```python
from build123d import *

# Parameters (mm, degrees)
SKETCH1_W                   = 15
SKETCH1_H                   = 4.9
SKETCH1_W_2                 = 5
SKETCH1_H_2                 = 19.05
SKETCH1_W_3                 = 14.05
BOSS_EXTRUDE1_DEPTH         = 30
SKETCH2_R                   = 6.4
CUT_EXTRUDE1_DEPTH          = 43.069832248
CUT_EXTRUDE2_DEPTH          = 30
FILLET1_R                   = 2.5
TAP_DRILL_FOR_M5X0_8_TAP1_D = 4.2


with BuildPart() as part:
    # Sketch1 → Boss-Extrude1 (new body)
    with BuildSketch(Plane(origin=(0, 0, 0), x_dir=(1, 0, 0), z_dir=(0, 1, 0))):
        with Locations((2.312030075, 14.354511278)):
            Rectangle(SKETCH1_W, SKETCH1_H)
        Polygon((-5.187969925, 16.804511278), (-10.187969925, 16.804511278), (-10.187969925, 11.329511278), (-5.187969925, 11.329511278), (-5.187969925, 11.904511278), align=None)
        with Locations((-7.687969925, 1.804511278)):
            Rectangle(SKETCH1_W_2, SKETCH1_H_2)
        with Locations((-17.212969925, 1.804511278)):
            Rectangle(SKETCH1_W_3, SKETCH1_H_2)
        Polygon((-5.187969925, -7.720488722), (-10.187969925, -7.720488722), (-10.187969925, -13.195488722), (-5.187969925, -13.195488722), (-5.187969925, -8.295488722), align=None)
        with Locations((2.312030075, -10.745488722)):
            Rectangle(SKETCH1_W, SKETCH1_H)
    extrude(amount=BOSS_EXTRUDE1_DEPTH)

    # Sketch2 → Cut-Extrude1 (cut, through all)
    with BuildSketch(Plane(origin=(0, 30, 0), x_dir=(1, 0, 0), z_dir=(0, 1, 0))):
        with Locations(Location((-14.712969925, 1.804511278, 0), (0, 0, 270))):
            Circle(SKETCH2_R)
    extrude(amount=-CUT_EXTRUDE1_DEPTH, mode=Mode.SUBTRACT)

    # Sketch4 → Cut-Extrude2 (cut)
    with BuildSketch(Plane(origin=(0, 30, 0), x_dir=(1, 0, 0), z_dir=(0, 1, 0))):
        with BuildLine():
            Line((-14.712969925, 11.329511278), (-24.237969925, 11.329511278))
            Line((-24.237969925, 11.329511278), (-24.237969925, 1.804511236))
            ThreePointArc((-24.237969925, 1.804511236), (-21.448162031, 8.539703354), (-14.712969925, 11.329511278))
        make_face()
        with BuildLine():
            ThreePointArc((-14.712969925, -7.720488722), (-21.448162001, -4.930680828), (-24.237969925, 1.804511236))
            Line((-24.237969925, 1.804511236), (-24.237969925, -7.720488722))
            Line((-24.237969925, -7.720488722), (-14.712969925, -7.720488722))
        make_face()
    extrude(amount=-CUT_EXTRUDE2_DEPTH, mode=Mode.SUBTRACT)

    # Fillet1
    fillet1_edges = [part.edges().sort_by_distance(p)[0] for p in [
        (-10.187969925, 15, 13.195488722),
        (-10.187969925, 15, 7.720488722),
        (-10.187969925, 15, -11.329511278),
        (-10.187969925, 15, -16.804511278),
    ]]
    fillet(fillet1_edges, radius=FILLET1_R)

    # Tap Drill for M5x0.8 Tap1 (through all)
    with Locations(Plane(origin=(0, 0, -16.804511278), x_dir=(-1, 0, 0), z_dir=(0, 0, -1))):
        with Locations((-2.312030075, 21.35), (-2.312030075, 8.65)):
            Hole(TAP_DRILL_FOR_M5X0_8_TAP1_D / 2)


solid = part.part
```
Read the model definition and answer for the solid it produces. Units are mm, in the model's axes. A direction names the side the tool comes from. Round coordinates to 2 decimals unless told otherwise and drop trailing zeros. Loops run counter-clockwise (first coordinate to the right, second up) from the corner with the lowest first, then second, coordinate; pieces in that order, holes last. Notation, with made-up numbers: (12, 17) -> (24, 17) arc R14 cw to (24, 22) -> close; hole circle Ø10 at (57.5, 12). An arc over 180 degrees is marked (long way). One line per item, written item: value.
1) Consider L1, parallel to Z at x = 0, y = 13.25; L2, parallel to X at y = 6.5, z = 2.5; L3, parallel to Z at x = -13, y = 19.25. Determine where each line is inside the solid, lowest interval first. Write a range as [from, to].
Answer list:
L1: z = [-16.8, -11.9], [8.3, 13.2]
L2: x = [-23.21, -19.45], [-9.98, -5.19]
L3: z = [-11.33, -7.97], [4.36, 7.72]
2) A cutting plane is placed at D-D (z = -6). Determine the outline of the cut face in (x, y), and give its area (3 significant figures).
Answer list:
outline: (-23.26, 0) -> (-19.55, 0) -> (-19.55, 30) -> (-23.26, 30) -> close; (-9.88, 0) -> (-5.19, 0) -> (-5.19, 30) -> (-9.88, 30) -> close
area: 252 mm²
3) A cutting plane is placed at C-C (y = 3.25). Determine the outline of the cut face in (x, z) (3 decimals).
Answer list:
outline: (-14.713, -11.33) -> (-12.688, -11.33) arc R2.5 cw to (-10.188, -13.83) -> (-10.188, -14.305) arc R2.5 ccw to (-7.688, -16.805) -> (9.812, -16.805) -> (9.812, -11.905) -> (-5.188, -11.905) -> (-5.188, 8.295) -> (9.812, 8.295) -> (9.812, 13.195) -> (-7.688, 13.195) arc R2.5 ccw to (-10.188, 10.695) -> (-10.188, 10.22) arc R2.5 cw to (-12.688, 7.72) -> (-14.713, 7.72) arc R9.525 ccw to start; hole circle Ø12.8 at (-14.713, -1.805)
4) For faces 1 (the face through (2, 15, 8.295)), 2 (the face through (-14, 15, -11.33)), 3 (the face through (1.86, 6.6, -14.32)), 4 (the face through (-14, 15, 7.72)), 5 (the face through (9.812, 15, -14)), determine the directions among +Z, -Z, +X, -X, +Y, -Y from which every point of the face is accessible in a straight line to the end or side of a thin tool.
Answer list:
face 1: +X, +Y, -Y
face 2: -Z, -X, +Y, -Y
face 3: +Z, -Z
face 4: +Z, -X, +Y, -Y
face 5: +Z, -Z, +X, +Y, -Y
5) A cutting plane is placed at A-A (y = 21.35). Determine the outline of the cut face in (x, z) (3 decimals).
Answer list:
outline: (-14.713, -11.33) -> (-12.688, -11.33) arc R2.5 cw to (-10.188, -13.83) -> (-10.188, -14.305) arc R2.5 ccw to (-7.688, -16.805) -> (0.212, -16.805) -> (0.212, -11.905) -> (-5.188, -11.905) -> (-5.188, 8.295) -> (0.212, 8.295) -> (0.212, 13.195) -> (-7.688, 13.195) arc R2.5 ccw to (-10.188, 10.695) -> (-10.188, 10.22) arc R2.5 cw to (-12.688, 7.72) -> (-14.713, 7.72) arc R9.525 ccw to start; (4.412, -16.805) -> (9.812, -16.805) -> (9.812, -11.905) -> (4.412, -11.905) -> close; (4.412, 8.295) -> (9.812, 8.295) -> (9.812, 13.195) -> (4.412, 13.195) -> close; hole circle Ø12.8 at (-14.713, -1.805)
6) The mould has two halves that part along Z. Classify faces 6 (the face through (1.86, 6.6, 10.78)), 7 (the face through (1, 15, 13.195)), 8 (the face through (-18.61, 15.21, -6.88)): pulls with the +Z half, pulls with the -Z half, needs draft (parallel to the pull), parting line crosses it, or undercut.
Answer list:
face 6: needs draft
face 7: pulls with the +Z half
face 8: undercut
7) A cutting plane is placed at B-B (x = 6.5). Determine the outline of the cut face in (y, z).
Answer list:
outline: (0, -16.8) -> (30, -16.8) -> (30, -11.9) -> (0, -11.9) -> close; (0, 8.3) -> (30, 8.3) -> (30, 13.2) -> (0, 13.2) -> close
8) Flat-ended cylindrical pins translate along their axes: P1, Ø6, axis at y = 9, z = 0.5, coming from the +X side; P2, Ø2.5, axis at x = 2.31, y = 8.65, coming from the +Z side; P3, Ø8, axis at y = 8.5, z = 7, coming from the -X side; P4, Ø0.5, axis at y = 16.5, z = 10.5, coming from the -X side. Find the tip coordinate at first contact, or state that the pin passes through.
Answer list:
P1: stops at x = -5.19
P2: passes through
P3: stops at x = -22.94
P4: stops at x = -10.19
